Can you work these out from the model? Positions are in its coordinate system, mm. Coordinates: 2 decimals unless noted, no trailing zeros. Loops run counter-clockwise (first coordinate to the right, second up) from the corner with the lowest first, then second, coordinate; pieces in that order, holes last. Notation, with made-up numbers: (65, 39) -> (79, 39) arc R20 cw to (79, 65) -> close; hole circle Ø2 at (-37.75, 36). An arc over 180 degrees is marked (long way). Use one line per item in the form item = value. Start each with the question number.
(1) I need wall thicknesses on line 1 (Y direction, x = 0, z = -13.5); line 2 (X direction, y = -33.5, z = -20.5); line 3 (X direction, y = -9, z = -7). Which ranges of each line are inside material? Lowest first, please. Write a range as [from, to].
(2) Imagine slicing it at A-A (z = -19.25). List the corners of the cut face in (x, y) for me.
(3) I'm going to push flat-ended pins straight in: pin 1 (8 mm diameter, centred on x = -94, z = -12.5, fed in from -Y); pin 2 (3 mm diameter, centred on y = 27, z = -8.5, fed in from -X); pin 3 (8 mm diameter, centred on x = 95, z = -7, fed in from -Y). Where does each tip first touch, or does it pass through?
(4) Imagine slicing it at B-B (x = 0). List the corners of the cut face in (y, z) for me.
(5) Imagine slicing it at C-C (x = 52). List the corners of the cut face in (y, z) for me, plus the area to 3 significant figures.
(6) Imagine slicing it at D-D (y = 6). List the corners of the cut face in (x, z) for me.
Solid Edge part; units mm, degrees
sketch "Sketch1" plane through (0, 0, 0) normal (0, 0, 1) x (1, 0, 0)
  line L0 (-120, -100) -> (120, -100)
  line L1 (120, -100) -> (120, 100)
  line L2 (120, 100) -> (-120, 100)
  line L3 (-120, 100) -> (-120, -100)
extrude "Protrusion1" add sketch "Sketch1" against normal blind 25
sketch "Sketch2" plane through (0, 0, -25) normal (0, 0, -1) x (-1, 0, 0)
  circle A0 centre (0, 30) radius 5
  line L0 (-100, 30) -> (-90, 30)
  arc A1 (-90, 30) -> (90, 30) centre (0, 30) ccw
  line L1 (90, 30) -> (100, 30)
  arc A2 (100, 30) -> (-100, 30) centre (0, 30) cw
extrude "ExtrudedCutout_2" cut sketch "Sketch2" against normal blind 25
sketch "Sketch3" plane through (0, 0, -25) normal (0, 0, -1) x (-1, 0, 0)
  line L0 (-115, 30.4369) -> (-120, 30.4369)
  line L1 (-120, 30.4369) -> (-120, -100)
  line L2 (-120, -100) -> (120, -100)
  line L3 (120, -100) -> (120, 30.4369)
  line L4 (120, 30.4369) -> (115, 30.4369)
  arc A0 (115, 30.4369) -> (-115, 30.4369) centre (0, 30.4369) cw
extrude "ExtrudedCutout_3" cut sketch "Sketch3" against normal blind 30
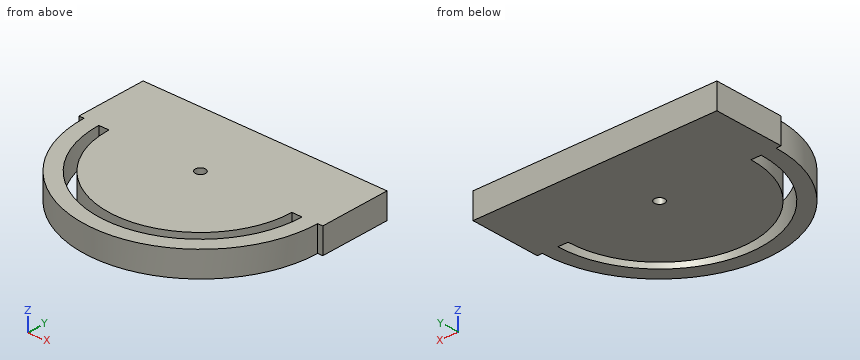
Worked out:
q1.line_1 = [-84.56, -70], [-60, 25], [35, 100]
q1.line_2 = [-95.59, -77.25], [-63.78, 63.78], [77.25, 95.59]
q1.line_3 = [-108.03, -92.08], [-81.11, 81.11], [92.08, 108.03]
q2.outline = (-120, 30.44) -> (-115, 30.44) arc R115 ccw to (115, 30.44) -> (120, 30.44) -> (120, 100) -> (-120, 100) -> close; hole (-100, 30) arc R100 ccw to (100, 30) -> (90, 30) arc R90 cw to (-90, 30) -> close; hole circle Ø10 at (0, 30)
q3.pin_1 = -41.15
q3.pin_2 = -114.98
q3.pin_3 = -39.88
q4.outline = (-84.56, -25) -> (-70, -25) -> (-70, 0) -> (-84.56, 0) -> close; (-60, -25) -> (25, -25) -> (25, 0) -> (-60, 0) -> close; (35, -25) -> (100, -25) -> (100, 0) -> (35, 0) -> close
q5.outline = (-72.14, -25) -> (-55.42, -25) -> (-55.42, 0) -> (-72.14, 0) -> close; (-43.46, -25) -> (100, -25) -> (100, 0) -> (-43.46, 0) -> close
q5.area = 4,000 mm2
q6.outline = (-112.37, -25) -> (-97.08, -25) -> (-97.08, 0) -> (-112.37, 0) -> close; (-86.74, -25) -> (86.74, -25) -> (86.74, 0) -> (-86.74, 0) -> close; (97.08, -25) -> (112.37, -25) -> (112.37, 0) -> (97.08, 0) -> close
